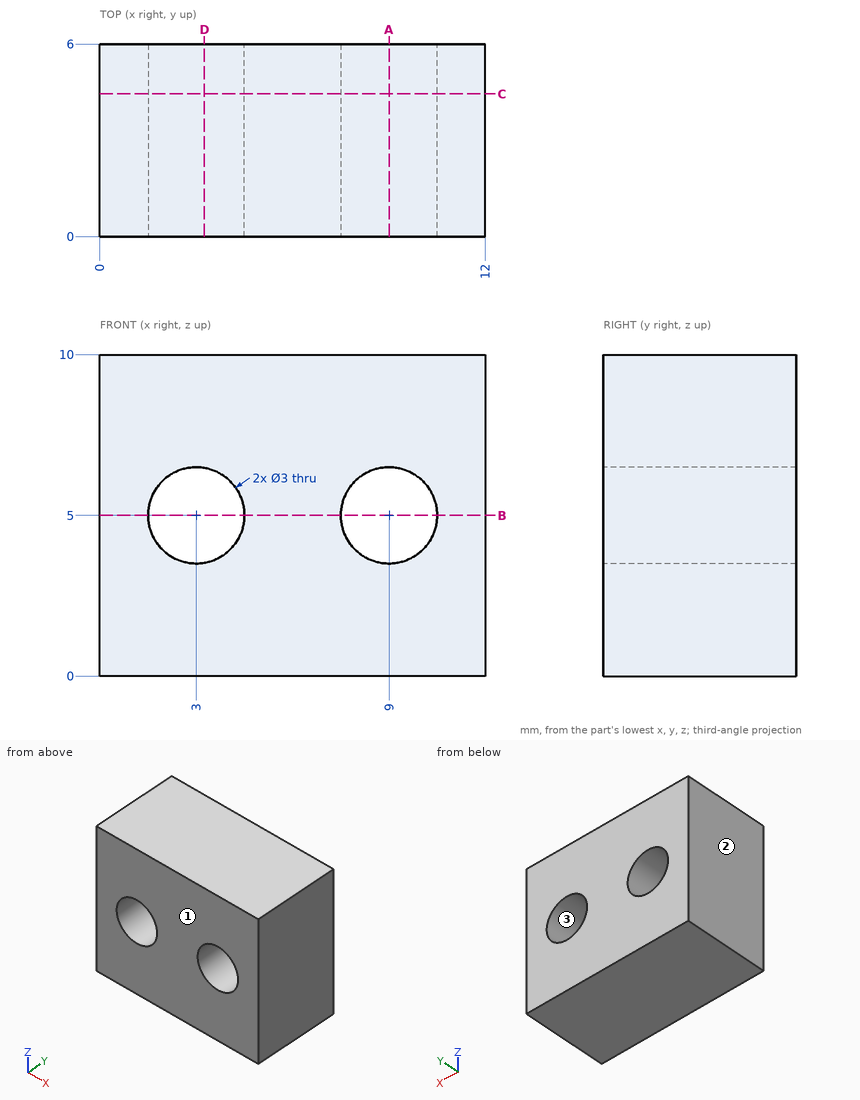
Study the drawing (mm; zero at the part's minimum x, y, z) and answer. Give positions to 0.01 mm unless a question says otherwise; leave off trailing zeros. Write each loop counter-clockwise with the first axis right and the second up, starting at its lowest first coordinate (ties: lowest second). Pieces come first, ordered by that corner, then holes.
Item 1: Section D-D, the plane x = 3.25 is taken. Write down the section's boundary in (y, z).
Item 2: Determine the mould class of the marked faces 1, 2 and 3 for opening direction X: released by +X, released by -X, zero draft, split by the parting line, or undercut.
Item 3: Section B-B, the plane z = 5 is taken. Write down the section's boundary in (x, y), plus the area to 3 significant figures.
Item 4: Section A-A, the plane x = 9 is taken. Write down the section's boundary in (y, z).
Item 5: A flat-ended cylindrical pin translates along its axis: P1, Ø3, axis at x = 5.5, z = 5.5, coming from the -Y side. Find the tip coordinate at first contact, or state that the pin passes through.
Item 6: Section C-C, the plane y = 4.45 is taken. Write down the section's boundary in (x, z), plus the area to 3 significant figures.
Item 7: Find the intervals of material crossed by line 1 along X through (y, z) = (1.2, 5); line 2 along Z through (x, y) = (3, 1.4); line 3 along X through (y, z) = (1.4, 4.5), in increasing order.
Completed:
1. outline: (0, 0) - (6, 0) - (6, 3.52) - (0, 3.52) - close; (0, 6.48) - (6, 6.48) - (6, 10) - (0, 10) - close
2. face 1: zero draft
2. face 2: released by -X
2. face 3: undercut
3. outline: (0, 0) - (1.5, 0) - (1.5, 6) - (0, 6) - close; (4.5, 0) - (7.5, 0) - (7.5, 6) - (4.5, 6) - close; (10.5, 0) - (12, 0) - (12, 6) - (10.5, 6) - close
3. area: 36.0 mm2
4. outline: (0, 0) - (6, 0) - (6, 3.5) - (0, 3.5) - close; (0, 6.5) - (6, 6.5) - (6, 10) - (0, 10) - close
5. P1: stops at y = 0
6. outline: (0, 0) - (12, 0) - (12, 10) - (0, 10) - close; hole circle Ø3 at (3, 5); hole circle Ø3 at (9, 5)
6. area: 106 mm2
7. line 1: x = 0 to 1.5, 4.5 to 7.5, 10.5 to 12
7. line 2: z = 0 to 3.5, 6.5 to 10
7. line 3: x = 0 to 1.59, 4.41 to 7.59, 10.41 to 12
